Source: CAD feature listing. Evaluate the final solid. Frame: model axes, mm. Face numbers are marked on the shaded views. A direction names the side the tool comes from. Round coordinates to 2 decimals unless told otherwise and drop trailing zeros. Write each loop counter-clockwise with the first axis right and the second up, starting at its lowest first coordinate (ties: lowest second). Pieces come first, ordered by that corner, then holes. Notation, with made-up numbers: M 43,64.5 L 53,64.5 A9 cw 53,71.5 Z; hole C 21,55.5 d8. An arc over 180 degrees is marked long. Answer in a Markdown table with one row per item.
from build123d import *

# Parameters (mm, degrees)
FILLET1_R                  = 0.7874
SKETCH2_W                  = 3.2639
SKETCH2_H                  = 20.6248
CUT_EXTRUDE1_DEPTH         = 8.9375
CUT_EXTRUDE1_DEPTH_BACK    = 8.9375
SKETCH3_R                  = 5.0038
SKETCH3_R_2                = 3.9624
CUT_EXTRUDE2_DEPTH         = 2.54
CHAMFER1_SIZE              = 0.762
SKETCH4_R                  = 3.97129
EXTRUDE1_DEPTH             = 11.176
CHAMFER2_SIZE              = 0.254
CHAMFER2_SIZE2             = 1.440505582
FILLET2_R                  = 1.524
EXTRUDE2_DEPTH             = 6.5
EXTRUDE2_DEPTH_BACK        = 6.5
CUT_EXTRUDE3_START         = 4.064
SKETCH6_R                  = 4.4958
CUT_EXTRUDE3_DEPTH         = 13.174
SKETCH7_R                  = 4.2545
EXTRUDE3_DEPTH             = 5.0038
CHAMFER3_SIZE              = 0.508
CUT_EXTRUDE4_DEPTH         = 3.9878
EXTRUDE4_REACH             = 19
SKETCH10_R                 = 2.5019
EXTRUDE4_DIRECTION_2_REACH = 19
SKETCH11_R                 = 15.875
SKETCH11_R_2               = 7.9375
EXTRUDE5_DEPTH             = 4.774946


with BuildPart() as part:
    # Sketch1 → Revolve1 (revolve)
    with BuildSketch(Plane(origin=(0, 0, 0), x_dir=(0, 0, -1), z_dir=(1, 0, 0))):
        Polygon((0, 30.3276), (7.9375, 30.3276), (7.9375, 1.3462), (5.0038, 1.3462), (5.0038, -9.8298), (0, -9.8298), align=None)
    revolve(axis=Axis((0, -15.35938, 0), (0, 1, 0)))

    # Fillet1
    fillet1_edges = [part.edges().sort_by_distance(p)[0] for p in [
        (0, 30.3276, 7.9375),
    ]]
    fillet(fillet1_edges, radius=FILLET1_R)

    # Sketch2 → Cut-Extrude1 (cut, two sides)
    with BuildSketch(Plane.XY) as cut_extrude1_sk:
        with Locations((6.30555, 20.0152)):
            Rectangle(SKETCH2_W, SKETCH2_H)
        with Locations((-6.30555, 20.0152)):
            Rectangle(SKETCH2_W, SKETCH2_H)
    extrude(amount=CUT_EXTRUDE1_DEPTH, mode=Mode.SUBTRACT)
    extrude(cut_extrude1_sk.sketch, amount=-CUT_EXTRUDE1_DEPTH_BACK, mode=Mode.SUBTRACT)

    # Sketch3 → Cut-Extrude2 (cut)
    with BuildSketch(Plane.XZ.offset(-1.3462)):
        with Locations(Location((0, 0, 0), (0, 0, 270))):  # turned: the seam where the file's is
            Circle(SKETCH3_R)
        with Locations(Location((0, 0, 0), (0, 0, 270))):  # turned: the seam where the file's is
            Circle(SKETCH3_R_2, mode=Mode.SUBTRACT)
    extrude(amount=CUT_EXTRUDE2_DEPTH, mode=Mode.SUBTRACT)

    # Chamfer1
    chamfer1_edges = [part.edges().sort_by_distance(p)[0] for p in [
        (0, -9.8298, 5.0038),
    ]]
    chamfer(chamfer1_edges, length=CHAMFER1_SIZE)

    # Sketch4 → Extrude1 (add, symmetric)
    with BuildSketch(Plane(origin=(0, 0, 0), x_dir=(0, 0, -1), z_dir=(1, 0, 0))):
        with Locations(Location((0, 20.8026, 0), (0, 0, 90))):  # turned: the seam where the file's is
            Circle(SKETCH4_R)
    extrude(amount=EXTRUDE1_DEPTH, both=True)

    # Chamfer2
    chamfer2_edges = [part.edges().sort_by_distance(p)[0] for p in [
        (11.176, 16.83131, 0),
    ]]
    chamfer2_side = [part.faces().sort_by_distance(p)[0] for p in [
        (11.176, 20.8026, 0),
    ]]
    chamfer(chamfer2_edges, length=CHAMFER2_SIZE, length2=CHAMFER2_SIZE2, reference=chamfer2_side[0])

    # Fillet2
    fillet2_edges = [part.edges().sort_by_distance(p)[0] for p in [
        (-11.176, 16.83131, 0),
    ]]
    fillet(fillet2_edges, radius=FILLET2_R)

    # Sketch5 → Extrude2 (add, two sides)
    with BuildSketch(Plane(origin=(0, 0, 0), x_dir=(1, 0, 0), z_dir=(0, 1, 0))) as extrude2_sk:
        with BuildLine():
            Line((7.900839338, 0.762), (16.982913649, 0.762))
            ThreePointArc((16.982913649, 0.762), (0, 17), (-16.982913649, 0.762))
            Line((-16.982913649, 0.762), (-7.900839338, 0.762))
            ThreePointArc((-7.900839338, 0.762), (0, 7.9375), (7.900839338, 0.762))
        make_face()
        with BuildLine():
            Line((7.900839338, -0.762), (16.982913649, -0.762))
            ThreePointArc((16.982913649, -0.762), (0, -17), (-16.982913649, -0.762))
            Line((-16.982913649, -0.762), (-7.900839338, -0.762))
            ThreePointArc((-7.900839338, -0.762), (0, -7.9375), (7.900839338, -0.762))
        make_face()
    extrude(amount=EXTRUDE2_DEPTH)
    extrude(extrude2_sk.sketch, amount=-EXTRUDE2_DEPTH_BACK)

    # Sketch6 → Cut-Extrude3 (cut, through all)
    with BuildSketch(Plane.XY.offset(0.762).offset(CUT_EXTRUDE3_START)):
        with Locations((12.2936, 0)):
            Circle(SKETCH6_R)
        with Locations((-12.2936, 0)):
            Circle(SKETCH6_R)
    extrude(amount=CUT_EXTRUDE3_DEPTH, mode=Mode.SUBTRACT)

    # Sketch7 → Extrude3 (add)
    with BuildSketch(Plane.XY.offset(4.826)):
        with Locations(Location((12.2936, 0, 0), (0, 0, 340.36075817))):  # turned: the seam where the file's is
            Circle(SKETCH7_R)
        with Locations(Location((-12.2936, 0, 0), (0, 0, 160.36075817))):  # turned: the seam where the file's is
            Circle(SKETCH7_R)
    extrude(amount=EXTRUDE3_DEPTH)

    # Chamfer3
    chamfer3_edges = [part.edges().sort_by_distance(p)[0] for p in [
        (8.286594981, 1.429923433, 9.8298),
        (-8.286594981, -1.429923433, 9.8298),
    ]]
    chamfer(chamfer3_edges, length=CHAMFER3_SIZE)

    # Sketch8 → Cut-Extrude4 (cut)
    with BuildSketch(Plane.XY.offset(9.8298)):
        Polygon((13.444778702, 1.9939), (14.595957403, 0), (13.444778702, -1.9939), (11.142421298, -1.9939), (9.991242597, 0), (11.142421298, 1.9939), align=None)
        Polygon((-14.595957403, 0), (-13.444778702, -1.9939), (-11.142421298, -1.9939), (-9.991242597, 0), (-11.142421298, 1.9939), (-13.444778702, 1.9939), align=None)
    extrude(amount=-CUT_EXTRUDE4_DEPTH, mode=Mode.SUBTRACT)

    # Sketch10 → Extrude4 (add, up to next)
    with BuildSketch(Plane.XY, mode=Mode.PRIVATE) as extrude4_sk1:
        with Locations((12.2936, 0)):
            Circle(SKETCH10_R)
    extrude4_tool1 = extrude(extrude4_sk1.sketch, amount=EXTRUDE4_REACH, mode=Mode.PRIVATE) - part.part
    add(extrude4_tool1.solids().sort_by_distance((12.2936, 0, 0))[0])
    # Sketch10 → Extrude4 (add, up to next)
    with BuildSketch(Plane.XY, mode=Mode.PRIVATE) as extrude4_sk2:
        with Locations((-12.2936, 0)):
            Circle(SKETCH10_R)
    extrude4_tool2 = extrude(extrude4_sk2.sketch, amount=EXTRUDE4_REACH, mode=Mode.PRIVATE) - part.part
    add(extrude4_tool2.solids().sort_by_distance((-12.2936, 0, 0))[0])

    # Sketch10 → Extrude4 direction 2 (add, up to next)
    with BuildSketch(Plane.XY, mode=Mode.PRIVATE) as extrude4_direction_2_sk1:
        with Locations((12.2936, 0)):
            Circle(SKETCH10_R)
    extrude4_direction_2_tool1 = extrude(extrude4_direction_2_sk1.sketch, amount=-EXTRUDE4_DIRECTION_2_REACH, mode=Mode.PRIVATE) - part.part
    add(extrude4_direction_2_tool1.solids().sort_by_distance((12.2936, 0, 0))[0])
    # Sketch10 → Extrude4 direction 2 (add, up to next)
    with BuildSketch(Plane.XY, mode=Mode.PRIVATE) as extrude4_direction_2_sk2:
        with Locations((-12.2936, 0)):
            Circle(SKETCH10_R)
    extrude4_direction_2_tool2 = extrude(extrude4_direction_2_sk2.sketch, amount=-EXTRUDE4_DIRECTION_2_REACH, mode=Mode.PRIVATE) - part.part
    add(extrude4_direction_2_tool2.solids().sort_by_distance((-12.2936, 0, 0))[0])

    # Sketch11 → Extrude5 (add)
    with BuildSketch(Plane(origin=(0, 6.5, 0), x_dir=(-1, 0, 0), z_dir=(0, 1, 0))):
        with Locations(Location((0, 0, 0), (0, 0, 182.751254589))):  # turned: the seam where the file's is
            Circle(SKETCH11_R)
        Circle(SKETCH11_R_2, mode=Mode.SUBTRACT)
    extrude(amount=EXTRUDE5_DEPTH)


solid = part.part
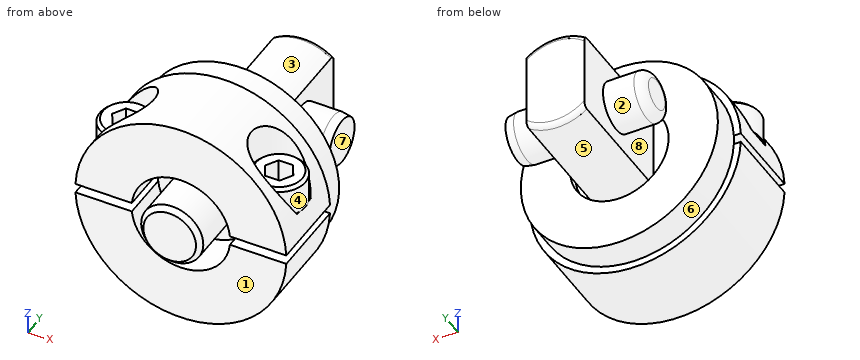
Q1. Section B-B (x = 0). Return loops of the section in (y, z) (1 decimal).
Solutions:
| item | result |
|---|---|
| outline | M -9.8,-4.2 L -9.1,-5 L -1.2,-5 L -1.2,-4 L 1.3,-4 L 1.3,-7.9 L -6.5,-7.9 L -6.5,-17 L 6.5,-17 L 6.5,-15.9 L 11.3,-15.9 L 11.3,-7.9 L 29.5,-7.9 A0.8 ccw 30.3,-7.2 L 30.3,7.2 A0.8 ccw 29.5,7.9 L 11.3,7.9 L 11.3,15.9 L 6.5,15.9 L 6.5,17 L -6.5,17 L -6.5,7.9 L 1.3,7.9 L 1.3,4 L -1.2,4 L -1.2,5 L -9.1,5 L -9.8,4.2 Z |
Q2. Material intervals for probe 1 along X at (y, z) = (0, 8.75); probe 2 along X at (y, z) = (0, 9.75); probe 3 along Y at (x, z) = (-11.5, 9), sorted ascending.
Solutions:
| item | result |
|---|---|
| probe 1 | x = -16.55 to -14.6, -9.99 to -8.04, -7.8 to 7.8, 8.04 to 9.99, 14.6 to 16.55 |
| probe 2 | x = -16.12 to -14.6, -9.99 to -8.47, -7.8 to 7.8, 8.47 to 9.99, 14.6 to 16.12 |
| probe 3 | y = -6.5 to -4.43, -4.18 to -1.99, 1.99 to 4.18, 4.43 to 11.27 |
Q3. Pull-direction query (Y, two-part tool) for the marked faces 1, 2 and 3; classes: pulls with the +Y half, pulls with the -Y half, needs draft (parallel to the pull), parting line crosses it, or undercut.
Solutions:
| item | result |
|---|---|
| face 1 | pulls with the -Y half |
| face 2 | undercut |
| face 3 | needs draft |
Q4. Access query for the marked faces 4, 5, 6, 7 and 8. Directions: +Z, -Z, +X, -X, +Y, -Y. A direction counts if a zero-diameter tool reaches every point of the face in a straight line with its end or side. Return the directions, or none.
Solutions:
| item | result |
|---|---|
| face 4 | +Z |
| face 5 | -Z, +Y |
| face 6 | +Y |
| face 7 | +Z, -Z, +X, +Y |
| face 8 | none |
Q5. Contact query for flat-ended pins moving along their axis: pin 1 Ø1.5 at (x, y) = (-9, 10) entering from +Z; pin 2 Ø0.5 at (x, z) = (-13, 0) entering from -Y; pin 3 Ø5.5 at (y, z) = (21, 1) entering from -X. Output: stop coordinate, or through.
Solutions:
| item | result |
|---|---|
| pin 1 | stops at z = 13.56 |
| pin 2 | stops at y = -2.46 |
| pin 3 | stops at x = -11.18 |
Q6. Section D-D (z = -14). Return loops of the section in (x, y), and give its area (3 significant figures).
Solutions:
| item | result |
|---|---|
| outline | M -9.64,-6.5 L 9.64,-6.5 L 9.64,6.5 L 7.48,6.5 L 7.48,11.27 L -7.48,11.27 L -7.48,6.5 L -9.64,6.5 Z |
| area | 322 mm2 |
